from build123d import *

# Parameters (mm, degrees)
ESQUISSE1_W             = 50
ESQUISSE1_H             = 45
BOSS_EXTRU_1_DEPTH      = 44.5
ESQUISSE2_W             = 40
ESQUISSE2_H             = 40
ENL_V_MAT_EXTRU_1_DEPTH = 44.5
ESQUISSE3_R             = 9.5
ESQUISSE3_R_2           = 1.5
ENL_V_MAT_EXTRU_2_DEPTH = 5
D_GAGEMENT_M31_D        = 3.4
CONG_1_R                = 15
ENL_V_MAT_EXTRU_3_REACH = 82.655
ESQUISSE7_R             = 3.25


with BuildPart() as part:
    # Esquisse1 → Boss.-Extru.1 (new body)
    with BuildSketch(Plane.XY):
        with Locations((25, 22.5)):
            Rectangle(ESQUISSE1_W, ESQUISSE1_H)
    extrude(amount=BOSS_EXTRU_1_DEPTH)

    # Esquisse2 → Enlèv. mat.-Extru.1 (cut)
    with BuildSketch(Plane.XY.offset(44.5)):
        with Locations((25, 25)):
            Rectangle(ESQUISSE2_W, ESQUISSE2_H)
    extrude(amount=-ENL_V_MAT_EXTRU_1_DEPTH, mode=Mode.SUBTRACT)

    # Esquisse3 → Enlèv. mat.-Extru.2 (cut)
    with BuildSketch(Plane(origin=(0, 5, 0), x_dir=(1, 0, 0), z_dir=(0, 1, 0))):
        with Locations(Location((33.25, -27.25, 0), (0, 0, 270))):
            Circle(ESQUISSE3_R)
        with Locations(Location((42.5, -18, 0), (0, 0, 270))):
            Circle(ESQUISSE3_R_2)
        with Locations(Location((24, -18, 0), (0, 0, 270))):
            Circle(ESQUISSE3_R_2)
        with Locations(Location((24, -36.5, 0), (0, 0, 270))):
            Circle(ESQUISSE3_R_2)
        with Locations(Location((42.5, -36.5, 0), (0, 0, 270))):
            Circle(ESQUISSE3_R_2)
    extrude(amount=-ENL_V_MAT_EXTRU_2_DEPTH, mode=Mode.SUBTRACT)

    # Dégagement M31 (through all)
    with Locations(Plane(origin=(0, 5, 0), x_dir=(1, 0, 0), z_dir=(0, 1, 0))):
        with Locations((42.5, -18), (24, -18), (24, -36.5), (42.5, -36.5)):
            Hole(D_GAGEMENT_M31_D / 2)

    # Congé1
    cong_1_edges = [part.edges().sort_by_distance(p)[0] for p in [
        (2.5, 45, 44.5),
        (47.5, 45, 44.5),
    ]]
    fillet(cong_1_edges, radius=CONG_1_R)

    # Enlèv. mat.-Extru.3: up to this face of the body (flat: up to its plane)
    enl_v_mat_extru_3_end = Plane(part.part.faces().sort_by_distance((0, 22.02684797, 21.783025057))[0])
    # Esquisse7 → Enlèv. mat.-Extru.3 (cut, up to the picked face)
    with BuildSketch(Plane(origin=(50, 0, 0), x_dir=(0, 0, -1), z_dir=(1, 0, 0)), mode=Mode.PRIVATE) as enl_v_mat_extru_3_sk1:
        with Locations((-27.25, 27.25)):
            Circle(ESQUISSE7_R)
    enl_v_mat_extru_3_tool1 = split(extrude(enl_v_mat_extru_3_sk1.sketch, amount=-ENL_V_MAT_EXTRU_3_REACH, mode=Mode.PRIVATE), bisect_by=enl_v_mat_extru_3_end, keep=Keep.BOTH, mode=Mode.PRIVATE)
    add(enl_v_mat_extru_3_tool1.solids().sort_by(Axis((50, 27.25, 27.25), (-1, 0, 0)))[0], mode=Mode.SUBTRACT)


solid = part.part
Work out the finished part from the listing and answer in its coordinate system (mm). A direction names the side the tool comes from. Give positions to 0.01 mm unless a question says otherwise; leave off trailing zeros. Loops run counter-clockwise (first coordinate to the right, second up) from the corner with the lowest first, then second, coordinate; pieces in that order, holes last. Notation, with made-up numbers: (26, 21) -> (81, 21) arc R14 cw to (81, 41) -> close; hole circle Ø2 at (75, 36). An arc over 180 degrees is marked (long way). Use a Markdown table: item, result. Add a question column.
1) This flat-tipped pin is pushed along its axis until it touches: P1, Ø1.5, axis at x = 23, z = 28, coming from the +Y side. Where does it stop, or does it pass through?
2) Which of the six approach directions +Z, -Z, +X, -X, +Y, -Y give full straight-line access (tool end or side, diameter ignored) to faces 4 (the cylindrical face through (43.85, 2.47, 37.53)), 5 (the flat face through (24.7, 5, 22.6))?
3) The part is cut by section D-D, the plane y = 27.25. Determine the outline of the cut face in (x, z).
4) Consider line 1 along X through (y, z) = (15.5, 12.5); line 2 along Y through (x, z) = (46.8, 27.25); line 3 along Y through (x, z) = (7.5, 2.5). Determine where each line is inside the solid, lowest interval first.
5) For a pull along X with two mould halves and no side action, classify faces 1 (the flat face through (50, 22, 22)), 2 (the cylindrical face through (23.2, 2.5, 38)), 3 (the flat face through (47, 45, 15)) as +X half, -X half, draft (parallel to the pull), parting line (faces both ways), or undercut.
6) The part is cut by section B-B, the plane x = 33.25. Determine the outline of the cut face in (y, z).
7) The part is cut by section A-A, the plane y = 9.5. Determine the outline of the cut face in (x, z).
8) The part is cut by section C-C, the plane z = 27.25. Determine the outline of the cut face in (x, y).
Reported:
| question | item | result |
|---|---|---|
| 1 | P1 | stops at y = 5 |
| 2 | face 4 | +Y, -Y |
| 2 | face 5 | +Z, -Z, +Y |
| 3 | outline | (0, 0) -> (5, 0) -> (5, 24) -> (0, 24) -> close; (0, 30.5) -> (5, 30.5) -> (5, 44.5) -> (0, 44.5) -> close; (45, 0) -> (50, 0) -> (50, 24) -> (45, 24) -> close; (45, 30.5) -> (50, 30.5) -> (50, 44.5) -> (45, 44.5) -> close |
| 4 | line 1 | x = 0 to 5, 45 to 50 |
| 4 | line 2 | y = 0 to 24, 30.5 to 45 |
| 4 | line 3 | y = 0 to 5 |
| 5 | face 1 | +X half |
| 5 | face 2 | undercut |
| 5 | face 3 | draft |
| 6 | outline | (0, 0) -> (5, 0) -> (5, 17.75) -> (0, 17.75) -> close; (0, 36.75) -> (5, 36.75) -> (5, 44.5) -> (0, 44.5) -> close |
| 7 | outline | (0, 0) -> (5, 0) -> (5, 44.5) -> (0, 44.5) -> close; (45, 0) -> (50, 0) -> (50, 44.5) -> (45, 44.5) -> close |
| 8 | outline | (0, 0) -> (23.75, 0) -> (23.75, 5) -> (5, 5) -> (5, 24) -> (0, 24) -> close; (0, 30.5) -> (5, 30.5) -> (5, 45) -> (0, 45) -> close; (42.75, 0) -> (50, 0) -> (50, 24) -> (45, 24) -> (45, 5) -> (42.75, 5) -> close; (45, 30.5) -> (50, 30.5) -> (50, 45) -> (45, 45) -> close |
